Part model, mm, in its own coordinate system. A direction names the side the tool comes from. Coordinates: 2 decimals unless noted, no trailing zeros. Order: outer loops, then holes, each group sorted by start corner. A loop starts at its lowest first (then second) coordinate and runs counter-clockwise, first axis right, second up.
1) Cut at C-C (y = 9.75). List the corners of the cut face in (x, z), and give its area (3 significant figures).
2) Tool access for faces 1 (the flat face through (224, 1.5, -8)), 2 (the flat face through (224, 7, 0)): list every direction of +Z, -Z, +X, -X, +Y, -Y with a clear straight run to the whole face (end or side of a thin tool).
3) Wall check: L1, parallel to Z at x = 437.5, y = 1.75; L2, parallel to Y at x = 225.5, z = -13.5. Give the ranges that are in metal, low to high.
4) Cut at B-B (z = -11.75). List the corners of the cut face in (x, y), and give its area (3 significant figures).
5) Cut at A-A (x = 189). List the corners of the cut face in (y, z).
6) Pin check, flat tips, straight feed: pin 1 Ø8 at (x, y) = (363, 3.5) entering from +Z; pin 2 Ø6 at (y, z) = (2, -4) entering from +X; pin 3 Ø4 at (y, z) = (1.5, -11) entering from +X; pin 4 Ø7 at (x, z) = (138, -11) entering from +Y. Stop position of each tip, or through.
```python
from build123d import *

# Parameters (mm, degrees)
EXTRUDE_1_DEPTH     = 455
CUT_EXTRUDE_1_DEPTH = 16


with BuildPart() as part:
    # Эскиз1 → Бобышка-Вытянуть1 (new body)
    with BuildSketch(Plane(origin=(0, 0, 0), x_dir=(0, 0, -1), z_dir=(1, 0, 0))):
        Polygon((0, 0), (0, 15), (1.5, 15), (1.5, 1.5), (15, 1.5), (15, 0), align=None)
    extrude(amount=EXTRUDE_1_DEPTH)

    # Эскиз2 → Вырез-Вытянуть1 (cut, through all)
    with BuildSketch(Plane.XZ):
        Polygon((455, 0), (434.173753179, -20.826246821), (455, -20.826246821), align=None)
    cut_extrude_1 = extrude(amount=-CUT_EXTRUDE_1_DEPTH, mode=Mode.SUBTRACT)

    # Зеркальное отражение1: Вырез-Вытянуть1 across plane
    add(cut_extrude_1.mirror(Plane(origin=(227.5, 0, 0), x_dir=(0, 0, 1), z_dir=(1, 0, 0))), mode=Mode.SUBTRACT)


solid = part.part
```
Geometry check:
1. outline: (0, 0) - (1.5, -1.5) - (453.5, -1.5) - (455, 0) - close
1. area: 680 mm2
2. face 1: -Z, +X, -X, +Y
2. face 2: +Z, +X, -X, +Y, -Y
3. L1: z = -1.5 to 0
3. L2: y = 0 to 1.5
4. outline: (11.75, 0) - (443.25, 0) - (443.25, 1.5) - (11.75, 1.5) - close
4. area: 647 mm2
5. outline: (0, -15) - (1.5, -15) - (1.5, -1.5) - (15, -1.5) - (15, 0) - (0, 0) - close
6. pin 1: stops at z = 0
6. pin 2: stops at x = 454
6. pin 3: stops at x = 446
6. pin 4: stops at y = 1.5
